Input: dimensioned drawing with shaded views. Units: mm. Origin: part minimum x, y, z. A direction names the side the tool comes from. Round coordinates to 2 decimals unless told otherwise and drop trailing zeros. Write each loop counter-clockwise with the first axis right and the second up, starting at its lowest first coordinate (ties: lowest second). Pieces come first, ordered by that corner, then holes. Notation, with made-up numbers: M -19.75,72.5 L 14.25,72.5 A33 ccw 14.25,109.5 Z; hole C 59,36 d11. An arc over 180 degrees is marked long. Put each result on its own line as item: value. Start each with the question number.
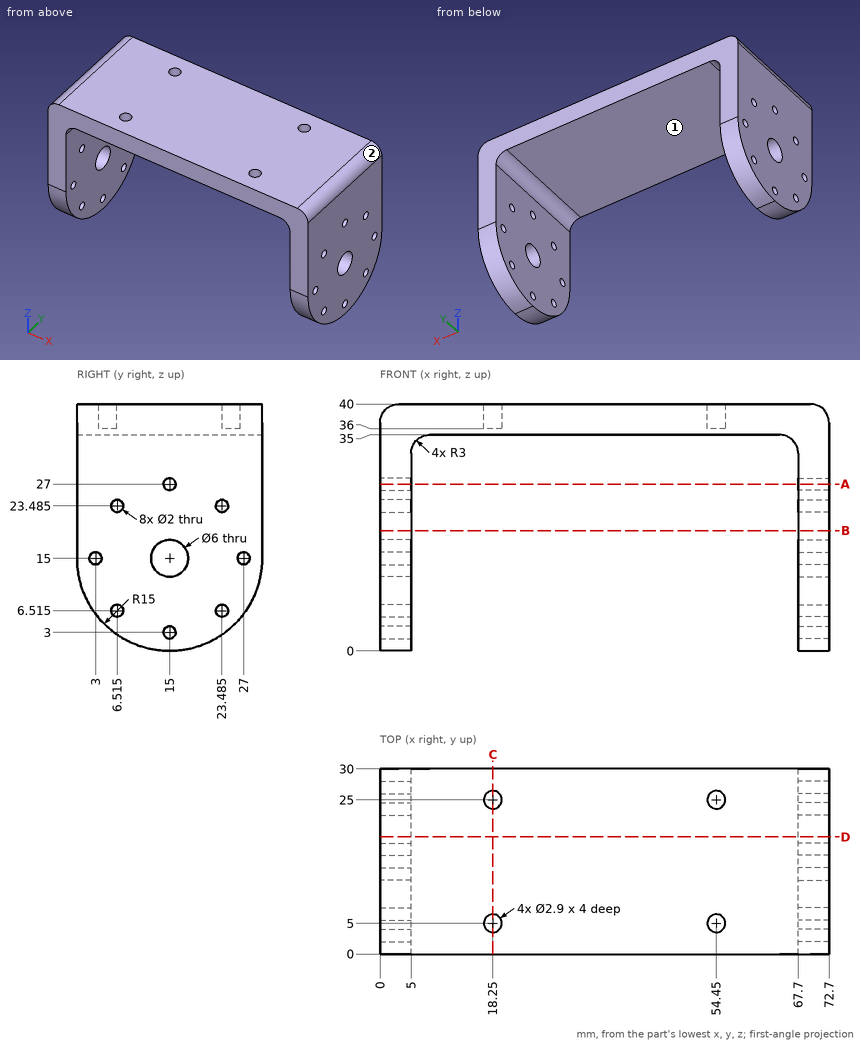
1) Ray query, probe 1 along Y at (x, z) = (1.45, 15); probe 2 along X at (y, z) = (9.5, 20); probe 3 along X at (y, z) = (23.75, 38) (1 decimal). Return the intervals inside material, ascending.
2) Section C-C, the plane x = 18.25. Output: boundary loops of the cut face in (y, z), and give its area (3 significant figures).
3) Section B-B, the plane z = 19.5. Output: boundary loops of the cut face in (x, y).
4) First-contact query: pin 1 (4 mm diameter, centred on x = 18.25, y = 25, fed in from -Z); pin 2 (2.5 mm diameter, centred on x = 18.25, y = 5, fed in from +Z). Flat tips, straight axial feed; report the tip coordinate or a pass-through.
5) Access query for the marked faces 1 and 2. Directions: +Z, -Z, +X, -X, +Y, -Y. A direction counts if a zero-diameter tool reaches every point of the face in a straight line with its end or side. Return the directions, or none.
6) Section A-A, the plane z = 27. Output: boundary loops of the cut face in (x, y), and give its area (3 significant figures).
7) Section D-D, the plane y = 19. Output: boundary loops of the cut face in (x, z).
Solved:
1. probe 1: y = 0 to 2, 4 to 12, 18 to 26, 28 to 30
1. probe 2: x = 0 to 5, 67.7 to 72.7
1. probe 3: x = 0.2 to 17.5, 19 to 53.7, 55.2 to 72.5
2. outline: M 0,35 L 30,35 L 30,40 L 26.45,40 L 26.45,36 L 23.55,36 L 23.55,40 L 6.45,40 L 6.45,36 L 3.55,36 L 3.55,40 L 0,40 Z
2. area: 127 mm2
3. outline: M 0,0 L 5,0 L 5,30 L 0,30 Z; M 67.7,0 L 72.7,0 L 72.7,30 L 67.7,30 Z
4. pin 1: stops at z = 35
4. pin 2: stops at z = 36
5. face 1: -Z, +Y, -Y
5. face 2: +Z, +X, +Y, -Y
6. outline: M 0,0 L 5,0 L 5,14 L 0,14 Z; M 0,16 L 5,16 L 5,30 L 0,30 Z; M 67.7,0 L 72.7,0 L 72.7,14 L 67.7,14 Z; M 67.7,16 L 72.7,16 L 72.7,30 L 67.7,30 Z
6. area: 280 mm2
7. outline: M 0,0.54 L 5,0.54 L 5,32 A3 cw 8,35 L 64.7,35 A3 cw 67.7,32 L 67.7,0.54 L 72.7,0.54 L 72.7,37 A3 ccw 69.7,40 L 3,40 A3 ccw 0,37 Z
